```python
from build123d import *

# Parameters (mm, degrees)
F1_DEPTH = 12.5
F2_W     = 10
F2_H     = 30
F3_DEPTH = 25
F4_W     = 10
F4_H     = 20
F5_DEPTH = 10
F6_R     = 5
F7_DEPTH = 25


with BuildPart() as f1:
    # F0 (on Front) → F1 (new body, symmetric)
    with BuildSketch(Plane.XZ):
        Polygon((-40, 0), (0, 0), (20, 200), (20, 250), (-40, 250), align=None)
    extrude(amount=F1_DEPTH, both=True)

    # F2 (on face) → F3 (cut)
    with BuildSketch(Plane.YZ.offset(20)):
        with Locations((0, 225)):
            Rectangle(F2_W, F2_H)
    extrude(amount=-F3_DEPTH, mode=Mode.SUBTRACT)

    # F4 (on face) → F5 (cut)
    with BuildSketch(Plane(origin=(0, 12.5, 0), x_dir=(-1, 0, 0), z_dir=(0, 1, 0))):
        with Locations((20, 100)):
            Rectangle(F4_W, F4_H)
    extrude(amount=-F5_DEPTH, mode=Mode.SUBTRACT)

    # F6 (on face) → F7 (cut)
    with BuildSketch(Plane.XY.offset(250)):
        with Locations((-25, 0)):
            Circle(F6_R)
    extrude(amount=-F7_DEPTH, mode=Mode.SUBTRACT)


solid = f1.part
```
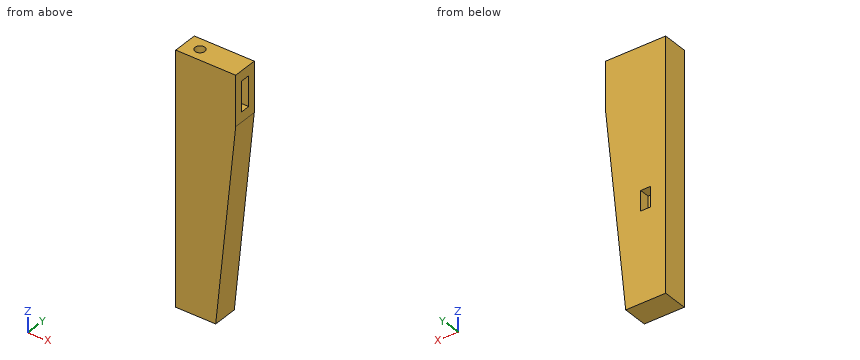
Model file for the job. Use its own axes, mm. Give positions to 0.01 mm unless a question says otherwise; leave off trailing zeros. Write each loop counter-clockwise with the first axis right and the second up, starting at its lowest first coordinate (ties: lowest second). Pieces come first, ordered by that corner, then holes. Notation, with made-up numbers: M 82.5,-25 L 122.5,-25 A18 cw 122.5,-8 Z; hole C 87.25,16.5 d9. An arc over 180 degrees is marked long. Use a Markdown table: item, result.
1) Cut at D-D (z = 144.5). List the corners of the cut face in (x, y), and give its area (3 significant figures).
Responses:
| item | result |
|---|---|
| outline | M -40,-12.5 L 14.45,-12.5 L 14.45,12.5 L -40,12.5 Z |
| area | 1,360 mm2 |
2) Pin check, flat tips, straight feed: pin 1 (6 mm diameter, centred on x = -25, y = 0, fed in from +Z); pin 2 (3 mm diameter, centred on x = -19, z = 104, fed in from +Y); pin 3 (11 mm diameter, centred on y = 10, z = 95.5, fed in from +X). Stop position of each tip, or through.
Responses:
| item | result |
|---|---|
| pin 1 | stops at z = 225 |
| pin 2 | stops at y = 2.5 |
| pin 3 | stops at x = 10.1 |
3) Drill centre lines: line 1 (Y direction, x = -25, z = 238.75); line 2 (Z direction, x = -3.5, y = 0); line 3 (X direction, y = -2, z = 67). Where is each one in solid material? Low to high. Write a range as from..to.
Responses:
| item | result |
|---|---|
| line 1 | y = -12.5..-5, 5..12.5 |
| line 2 | z = 0..210, 240..250 |
| line 3 | x = -40..6.7 |
4) Cut at B-B (x = 5). List the corners of the cut face in (y, z).
Responses:
| item | result |
|---|---|
| outline | M -12.5,50 L 12.5,50 L 12.5,250 L -12.5,250 Z; hole M -5,210 L 5,210 L 5,240 L -5,240 Z |
5) Cut at C-C (y = 0). List the corners of the cut face in (x, z), and give its area (3 significant figures).
Responses:
| item | result |
|---|---|
| outline | M -40,0 L 0,0 L 20,200 L 20,210 L -5,210 L -5,240 L 20,240 L 20,250 L -20,250 L -20,225 L -30,225 L -30,250 L -40,250 Z |
| area | 12,000 mm2 |
6) Cut at A-A (y = 9.5). List the corners of the cut face in (x, z).
Responses:
| item | result |
|---|---|
| outline | M -40,0 L 0,0 L 20,200 L 20,250 L -40,250 Z; hole M -25,90 L -15,90 L -15,110 L -25,110 Z |
